For this review, take the finished solid that the model builds, in its own axes (mm). Face numbers are marked on the shaded views. Give positions to 0.01 mm unless a question says otherwise; leave off trailing zeros. Loops run counter-clockwise (first coordinate to the right, second up) from the corner with the lowest first, then second, coordinate; pieces in that order, holes last. Notation, with made-up numbers: (72.25, 13) -> (112.25, 13) arc R26 ccw to (112.25, 29) -> close; hole circle Ø3 at (61, -25.75). An arc over 180 degrees is marked (long way). One line per question, with ' | ' between items. Start each with the question number.
(1) Wall thickness on probe 1 along X at (y, z) = (-1, 0) (3 decimals); probe 2 along Z at (x, y) = (-0.05, -4); probe 3 along Z at (x, y) = (-0.3, -2.25): over which ranges is each line inside the solid? List them lowest first.
(2) Insertion check: P1, Ø2, axis at y = -3, z = -1.5, coming from the +X side; P2, Ø2, axis at x = 0, y = -1, coming from the -Z side (3 decimals). Each pin has a flat end and moves straight along its axis. Give the tip position at first contact, or say it passes through.
(3) Consider section B-B (z = 0). Write out the cut boundary in (x, y) (3 decimals).
(4) Draft analysis for pull direction Z (two halves, no side actions). For the marked faces 1, 2 and 3, state which applies: +Z half, -Z half, draft (parallel to the pull), parting line (faces both ways), or undercut.
(5) Consider section A-A (x = 0). Write out the cut boundary in (y, z) (3 decimals).
(6) Consider section C-C (y = -1.5). Write out the cut boundary in (x, z) (3 decimals).
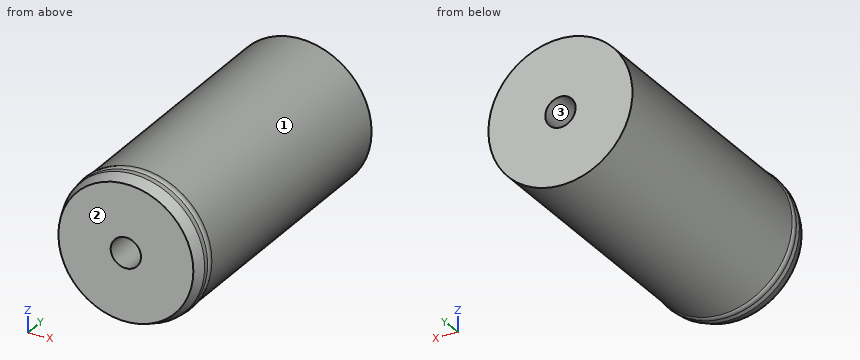
from build123d import *

# Parameters (mm, degrees)
SKETCH013_R         = 2.115
SKETCH013_R_2       = 0.445
PAD006_DEPTH        = 7
SKETCH015_R         = 0.225
GROOVE001_FACE2_R   = 2.115
GROOVE001_FACE2_R_2 = 0.445
PAD007_DEPTH        = 0.2
PAD007_FACE5_R      = 2.115
PAD007_FACE5_R_2    = 0.445
PAD008_DEPTH        = 1.6


with BuildPart() as part:
    # Sketch013 → Pad006 (new body)
    with BuildSketch(Plane.XZ):
        Circle(SKETCH013_R)
        Circle(SKETCH013_R_2, mode=Mode.SUBTRACT)
    extrude(amount=PAD006_DEPTH)

    # Sketch015 → Revolution (revolve)
    with BuildSketch(Plane.XY):
        with Locations((-1.916694, -6.398077)):
            Circle(SKETCH015_R)
    revolve(axis=Axis((0, 0, 0), (0, 1, 0)))

    # Sketch016 → Groove001 (revolve, cut)
    with BuildSketch(Plane.XY):
        Polygon((-2.238852, -6.34167), (-1.80714, -7.444808), (-2.2822, -7.159883), align=None)
    revolve(axis=Axis((0, 0, 0), (0, 1, 0)), mode=Mode.SUBTRACT)

    # Groove001 Face2 → Pad007 (add)
    with BuildSketch(Plane(origin=(0, 0, 0), x_dir=(1, 0, 0), z_dir=(0, 1, 0))):
        Circle(GROOVE001_FACE2_R)
        Circle(GROOVE001_FACE2_R_2, mode=Mode.SUBTRACT)
    extrude(amount=PAD007_DEPTH)

    # Pad007 Face5 → Pad008 (add)
    with BuildSketch(Plane(origin=(0, 0.2, 0), x_dir=(1, 0, 0), z_dir=(0, 1, 0))):
        Circle(PAD007_FACE5_R)
        Circle(PAD007_FACE5_R_2, mode=Mode.SUBTRACT)
    extrude(amount=PAD008_DEPTH)


solid = part.part
A:
1) probe 1: x = -2.115 to -0.445, 0.445 to 2.115 | probe 2: z = -2.11 to -0.44, 0.44 to 2.11 | probe 3: z = -2.09 to -0.33, 0.33 to 2.09
2) P1: stops at x = 2.06 | P2: stops at z = -2.115
3) outline: (-2.115, -6.658) -> (-1.981, -7) -> (-0.445, -7) -> (-0.445, 1.8) -> (-2.115, 1.8) -> (-2.115, -6.292) arc R0.225 ccw to (-2.115, -6.504) -> close; (0.445, -7) -> (1.981, -7) -> (2.115, -6.658) -> (2.115, -6.504) arc R0.225 ccw to (2.115, -6.292) -> (2.115, 1.8) -> (0.445, 1.8) -> close
4) face 1: parting line | face 2: draft | face 3: undercut
5) outline: (-7, -1.981) -> (-6.658, -2.115) -> (-6.504, -2.115) arc R0.225 ccw to (-6.292, -2.115) -> (1.8, -2.115) -> (1.8, -0.445) -> (-7, -0.445) -> close; (-7, 0.445) -> (1.8, 0.445) -> (1.8, 2.115) -> (-6.292, 2.115) arc R0.225 ccw to (-6.504, 2.115) -> (-6.658, 2.115) -> (-7, 1.981) -> close
6) outline: circle Ø4.23 at (0, 0); hole circle Ø0.89 at (0, 0)
